Read the model definition and answer for the solid it produces. Units are mm, in the model's axes. A direction names the side the tool comes from. Coordinates: 2 decimals unless noted, no trailing zeros. Order: outer loops, then holes, each group sorted by start corner. A loop starts at its lowest first (then second) coordinate and runs counter-clockwise, first axis right, second up. Notation, with made-up numbers: (11, 85) -> (68, 85) arc R20 ccw to (68, 108) -> close; hole circle Ø7 at (24, 70). An arc over 180 degrees is marked (long way). Answer in a Markdown table with one row per item.
Autodesk Inventor part; units mm, degrees
ref_plane "YZ Plane" through (0, 0, 0) normal (1, 0, 0) x (0, 1, 0)
ref_plane "XZ Plane" through (0, 0, 0) normal (0, 1, 0) x (-1, 0, 0)
ref_plane "XY Plane" through (0, 0, 0) normal (0, 0, 1) x (1, 0, 0)
sketch "スケッチ1" plane through (0, 0, 0) normal (0, 0, 1) x (1, 0, 0)
  line L0 (0, 0) -> (-17.6777, 17.6777)
  line L1 (-17.6777, 17.6777) -> (17.6777, 17.6777)
  line L2 (17.6777, 17.6777) -> (0, 0)
  line L3 (-17.6777, 17.6777) -> (-21.2487, 14.1066)
  line L4 (0, 0) -> (-2.2909, -2.2909)
  circle A0 centre (-10.435, 14.6777) radius 0.8
  circle A1 centre (10.435, 14.6777) radius 0.8
  circle A2 centre (0, 4.2426) radius 0.8
  dimension "d0" = 25
  dimension "d1" = 45
  dimension "d5" = 1.6
  dimension "d6" = 1.6
  dimension "d7" = 1.6
  dimension "d8" = 3
  dimension "d9" = 3
  dimension "d10" = 3
  dimension "d11" = 3
  dimension "d12" = 3
  dimension "d13" = 3
extrude "押し出し1" add sketch "スケッチ1" along normal blind 26
fillet "フィレット1" radius 2 3 edges at (17.6777, 17.6777, 13) (0, 0, 13) (-17.6777, 17.6777, 13)
sketch "スケッチ2" plane through (-12.8492, 17.6777, 0) normal (0, 1, 0) x (1, 0, 0)
  line L0 (0, -26) -> (0, 0)
  line L1 (25.6985, -26) -> (0, -26)
  line L2 (25.6985, 0) -> (25.6985, -26)
  line L3 (25.6985, 0) -> (0, 0)
  line L4 (25.6985, -26) -> (0, 0)
  line L5 (0, -26) -> (-2, -26)
  line L6 (0, -26) -> (25.6985, 0)
  circle A0 centre (12.8492, -13) radius 4.25
  circle A1 centre (12.8492, -13) radius 6 construction
  circle A2 centre (12.8492, -19) radius 0.8
  circle A3 centre (17.0919, -17.2426) radius 0.8
  circle A4 centre (18.8492, -13) radius 0.8
  circle A5 centre (17.0919, -8.7574) radius 0.8
  circle A6 centre (12.8492, -7) radius 0.8
  circle A7 centre (8.6066, -8.7574) radius 0.8
  circle A8 centre (12.8492, -13) radius 8
  circle A9 centre (6.8492, -13) radius 0.8
  circle A10 centre (8.6066, -17.2426) radius 0.8
  point P0 (12.8492, 0)
  point P1 (-1.4142, -26)
  dimension "d15" = 12
  dimension "d14" = 8.5
  dimension "d16" = 1.6
  dimension "d23" = 360
  dimension "d25" = 16
extrude "押し出し2" cut sketch "スケッチ2" against normal through all contours A8 L4 A7 A0 L6 A10 | L6 A10 A0 L4 A3 A8 | A8 L6 A5 A0 L4 A7 | L4 A3 A0 L6 A5 A8 | A10 L6 | L6 A10 | A7 L4 | L4 A7 | A3 L4 | L4 A3 | A5 L6 | L6 A5 | A0 L4 L6 | L6 L4 A0 | A0 L6 L4 | L4 L6 A0 | A2 | A4 | A6 | A9
extrude "押し出し3" add sketch "スケッチ2" against normal blind 1.5 contours A8 L4 A7 A0 L6 A10 | L6 A10 A0 L4 A3 A8 | A8 L6 A5 A0 L4 A7 | L4 A3 A0 L6 A5 A8
sketch "スケッチ4" plane through (0, 0, 26) normal (0, 0, 1) x (1, 0, 0)
  line L0 (-4.2929, 7.1213) -> (-7.6066, 10.435)
  arc A0 (-7.6066, 14.6777) -> (-7.6066, 10.435) centre (-5.4853, 12.5563) ccw
  arc A1 (-5.364, 15.6777) -> (-7.4853, 14.799) centre (-5.364, 12.6777) ccw
  line L1 (-7.6066, 14.6777) -> (-7.4853, 14.799)
  line L2 (-5.364, 15.6777) -> (5.364, 15.6777)
  arc A2 (7.4853, 14.799) -> (5.364, 15.6777) centre (5.364, 12.6777) ccw
  arc A3 (7.6066, 10.435) -> (7.6066, 14.6777) centre (5.4853, 12.5563) ccw
  line L3 (7.4853, 14.799) -> (7.6066, 14.6777)
  line L4 (7.6066, 10.435) -> (4.2929, 7.1213)
  arc A4 (2.1716, 6.2426) -> (4.2929, 7.1213) centre (2.1716, 9.2426) ccw
  line L5 (2.1716, 6.2426) -> (-2.1716, 6.2426)
  arc A5 (-4.2929, 7.1213) -> (-2.1716, 6.2426) centre (-2.1716, 9.2426) ccw
  point P0 (0, 0)
extrude "押し出し5" cut sketch "スケッチ4" against normal blind 21
equation "\"d9\" = d8"
equation "\"d10\" = d8"
equation "\"d11\" = d8"
equation "\"d12\" = d8"
equation "\"d13\" = d8"
equation "\"BendRadius\" = Thickness"
equation "\"BendReliefWidth\" = Thickness"
equation "\"BendReliefDepth\" = 0.5 * Thickness"
equation "\"CornerReliefSize\" = 4 * Thickness"
equation "\"MinimumRemnant\" = 2 * Thickness"
equation "\"TransitionRadius\" = BendRadius"
equation "\"JacobiRadiusSize\" = BendRadius"
equation "\"GapSize\" = Thickness"
properties part number "hipjoint_middle"
Q1. For faces 1 (the face through (3.4, 16.178, 16.4)), 2 (the face through (3.304, 6.465, 22.919)), 3 (the face through (10.8, 15.39, 12.82)), determine the directions among +Z, -Z, +X, -X, +Y, -Y from which every point of the face is accessible in a straight line to the end or side of a thin tool.
Outcome:
| item | result |
|---|---|
| face 1 | -Y |
| face 2 | +Z |
| face 3 | +Z, -Z |
Q2. Consider line 1 (Z direction, x = 0, y = 16.8); line 2 (X direction, y = 15, z = 6.5); line 3 (X direction, y = 17.1, z = 13). Determine where each line is inside the solid, lowest interval first.
Outcome:
| item | result |
|---|---|
| line 1 | 0 to 6.2, 7.8 to 8.75, 17.25 to 18.2, 19.8 to 26 |
| line 2 | -14.73 to -11.17, -9.7 to -7.26, 7.26 to 9.7, 11.17 to 14.73 |
| line 3 | -14.26 to -6.8, -5.2 to -4.25, 4.25 to 5.2, 6.8 to 14.26 |
Q3. The part is cut by section C-C (y = 2). Write down the section's boundary in (x, z).
Outcome:
| item | result |
|---|---|
| outline | (-2, 0) -> (2, 0) -> (2, 5.25) arc R8 cw to (-2, 5.25) -> close; (-2, 20.75) arc R8 cw to (2, 20.75) -> (2, 26) -> (-2, 26) -> close |
Q4. The part is cut by section A-A (z = 13). Write down the section's boundary in (x, y) (3 decimals), then the cut area to 3 significant figures.
Outcome:
| item | result |
|---|---|
| outline | (-14.263, 14.263) -> (-8, 8) -> (-8, 10.92) arc R3 cw to (-8, 14.192) -> (-8, 16.178) -> (-6.8, 16.178) -> (-6.8, 17.678) -> (-12.849, 17.678) arc R2 ccw to start; (-5.2, 16.178) -> (-4.25, 16.178) -> (-4.25, 17.678) -> (-5.2, 17.678) -> close; (4.25, 16.178) -> (5.2, 16.178) -> (5.2, 17.678) -> (4.25, 17.678) -> close; (6.8, 16.178) -> (8, 16.178) -> (8, 14.192) arc R3 cw to (8, 10.92) -> (8, 8) -> (14.263, 14.263) arc R2 ccw to (12.849, 17.678) -> (6.8, 17.678) -> close; hole circle Ø1.6 at (-10.435, 14.678); hole circle Ø1.6 at (10.435, 14.678) |
| area | 84.0 mm² |
Q5. Given pin 1 (2.5 mm diameter, centred on x = -10.44, y = 14.68, fed in from +Z); pin 2 (1.7 mm diameter, centred on x = 4, z = 6.5, fed in from -Y); pin 3 (6 mm diameter, centred on y = 11, z = 5.5, fed in from +X); pin 4 (2 mm diameter, centred on x = 10.5, z = 12, fed in from -Y), each flat-ended and moving along its own axis, determine where each tip first touches the part or whether it passes through.
Outcome:
| item | result |
|---|---|
| pin 1 | z = 26 |
| pin 2 | y = 3.51 |
| pin 3 | x = 14 |
| pin 4 | y = 9.5 |
Q6. For a pull along X with two mould halves and no side action, classify faces 4 (the face through (9, 9, 13)), 5 (the face through (0, 11, 0)), 6 (the face through (-4.347, 16.938, 7.964)) as pulls with the +X half, pulls with the -X half, needs draft (parallel to the pull), parting line crosses it, or undercut.
Outcome:
| item | result |
|---|---|
| face 4 | pulls with the +X half |
| face 5 | needs draft |
| face 6 | undercut |
Q7. The part is cut by section D-D (z = 2.75). Write down the section's boundary in (x, y) (3 decimals), then the cut area to 3 significant figures.
Outcome:
| item | result |
|---|---|
| outline | (-14.263, 14.263) -> (-1.414, 1.414) arc R2 ccw to (1.414, 1.414) -> (14.263, 14.263) arc R2 ccw to (12.849, 17.678) -> (-12.849, 17.678) arc R2 ccw to start; hole circle Ø1.6 at (-10.435, 14.678); hole circle Ø1.6 at (0, 4.243); hole circle Ø1.6 at (10.435, 14.678) |
| area | 296 mm² |
Q8. The part is cut by section B-B (x = 6). Write down the section's boundary in (y, z).
Outcome:
| item | result |
|---|---|
| outline | (6, 0) -> (17.68, 0) -> (17.68, 12.2) -> (16.18, 12.2) -> (16.18, 7.71) -> (15.61, 7.71) -> (15.61, 5) -> (8.83, 5) -> (8.83, 7.71) -> (6, 7.71) -> close; (6, 18.29) -> (8.83, 18.29) -> (8.83, 26) -> (6, 26) -> close; (15.61, 18.29) -> (16.18, 18.29) -> (16.18, 13.8) -> (17.68, 13.8) -> (17.68, 26) -> (15.61, 26) -> close |
